```python
from build123d import *

# Parameters (mm, degrees)
F1_DEPTH = 15
F2_R     = 2.8
F3_DEPTH = 45.401
F4_R     = 5


with BuildPart() as f1:
    # F0 (on Front) → F1 (new body)
    with BuildSketch(Plane.XZ):
        with BuildLine():
            ThreePointArc((-11.5, 0), (0, 11.5), (11.5, 0))
            Line((11.5, 0), (11.5, -10))
            Line((11.5, -10), (22.7, -10))
            Line((22.7, -10), (22.7, 0))
            Line((22.7, 0), (22.7, 17.013083))
            Line((22.7, 17.013083), (6.196252, 17.013083))
            ThreePointArc((6.196252, 17.013083), (0, 19.79383), (-6.196252, 17.013083))
            Line((-6.196252, 17.013083), (-22.7, 17.013083))
            Line((-22.7, 17.013083), (-22.7, 0))
            Line((-22.7, 0), (-22.7, -10))
            Line((-22.7, -10), (-11.5, -10))
            Line((-11.5, -10), (-11.5, 0))
        make_face()
    extrude(amount=F1_DEPTH)

    # F2 (on face) → F3 (cut, through all)
    with BuildSketch(Plane.YZ.offset(22.7)):
        with Locations((-7.5, 0)):
            Circle(F2_R)
    extrude(amount=-F3_DEPTH, mode=Mode.SUBTRACT)

    # F4
    f4_edges = [f1.edges().sort_by_distance(p)[0] for p in [
        (6.196252, -7.5, 17.013083),
        (-6.196252, -7.5, 17.013083),
    ]]
    fillet(f4_edges, radius=F4_R)


solid = f1.part
```
Can you work these out from the model? Positions are in its coordinate system, mm. A direction names the side the tool comes from. Round coordinates to 2 decimals unless told otherwise and drop trailing zeros. Loops run counter-clockwise (first coordinate to the right, second up) from the corner with the lowest first, then second, coordinate; pieces in that order, holes last. Notation, with made-up numbers: M -37,-25 L 9,-25 A19 ccw 9,-2 Z; hole C -35.75,44.5 d1. An arc over 180 degrees is marked long. Answer in a Markdown table with one row per item.
1. Thinking about a two-plate mould opening in X: for faces 1 (the face through (22.7, -7, 3)), 2 (the face through (-15, -7, 17.013)), 3 (the face through (-11.5, -7, -5)), which applies, pulls with the +X half, pulls with the -X half, needs draft (parallel to the pull), parting line crosses it, or undercut?
Established:
| item | result |
|---|---|
| face 1 | pulls with the +X half |
| face 2 | needs draft |
| face 3 | undercut |
2. On a 3-axis mill with a long thin cutter (end or side, diameter ignored), from which of +Z, -Z, +X, -X, +Y, -Y can I reach the whole of each face in a straight line? I mean faces 4 (the face through (16, -7, 17.013)), 5 (the face through (-17, -7, -10)), 6 (the face through (11.5, -7, -5)). Say none if no direction works.
Established:
| item | result |
|---|---|
| face 4 | +Z, +X, +Y, -Y |
| face 5 | -Z, +X, -X, +Y, -Y |
| face 6 | -Z, +Y, -Y |
3. If we section it at D-D, the plane y = -3.25: Please give me the cut outline in (x, z).
Established:
| item | result |
|---|---|
| outline | M -22.7,-10 L -11.5,-10 L -11.5,0 A11.5 cw 11.5,0 L 11.5,-10 L 22.7,-10 L 22.7,17.01 L 8.14,17.01 A5 cw 5.08,18.06 A8.29 ccw -5.08,18.06 A5 cw -8.14,17.01 L -22.7,17.01 Z |
4. If we section it at C-C, the plane x = 13: Please give me the cut outline in (y, z), plus the area to 3 significant figures.
Established:
| item | result |
|---|---|
| outline | M -15,-10 L 0,-10 L 0,17.01 L -15,17.01 Z; hole C -7.5,0 d5.6 |
| area | 381 mm² |
5. Please list where these lines run through material, in increasing order: line 1 (X direction, y = -9.25, z = -3.5); line 2 (Z direction, x = -20, y = -7.5); line 3 (X direction, y = -8.25, z = 6.5). Write a range as from..to.
Established:
| item | result |
|---|---|
| line 1 | -22.7..-11.5, 11.5..22.7 |
| line 2 | -10..-2.8, 2.8..17.01 |
| line 3 | -22.7..-9.49, 9.49..22.7 |
6. If we section it at B-B, the plane y = -7.5: Please give me the cut outline in (x, z), plus the area to 3 significant figures.
Established:
| item | result |
|---|---|
| outline | M -22.7,-10 L -11.5,-10 L -11.5,-2.8 L -22.7,-2.8 Z; M -22.7,2.8 L -11.15,2.8 A11.5 cw 11.15,2.8 L 22.7,2.8 L 22.7,17.01 L 8.14,17.01 A5 cw 5.08,18.06 A8.29 ccw -5.08,18.06 A5 cw -8.14,17.01 L -22.7,17.01 Z; M 11.5,-10 L 22.7,-10 L 22.7,-2.8 L 11.5,-2.8 Z |
| area | 687 mm² |
7. I'm going to push flat-ended pins straight in: pin 1 Ø6 at (x, y) = (9.5, -11.5) entering from +Z; pin 2 Ø8 at (x, y) = (-13, -9) entering from +Z. Where does each tip first touch, or does it pass through?
Established:
| item | result |
|---|---|
| pin 1 | z = 17.29 |
| pin 2 | z = 17.01 |
8. If we section it at A-A, the plane z = -4: Please give me the cut outline in (x, y).
Established:
| item | result |
|---|---|
| outline | M -22.7,-15 L -11.5,-15 L -11.5,0 L -22.7,0 Z; M 11.5,-15 L 22.7,-15 L 22.7,0 L 11.5,0 Z |
